Source: CAD feature listing. Evaluate the final solid. Frame: model axes, mm. A direction names the side the tool comes from. Give positions to 0.01 mm unless a question says otherwise; leave off trailing zeros. Write each loop counter-clockwise with the first axis right and the second up, starting at its lowest first coordinate (ties: lowest second). Pieces come first, ordered by that corner, then holes. Notation, with made-up numbers: M 26.5,-9.5 L 30.5,-9.5 A20 ccw 30.5,1.5 Z; hole C -39,38.5 d4. An arc over 180 degrees is marked long. Return JSON: item names as keys, results as strings.
```python
from build123d import *

# Parameters (mm, degrees)
SKETCH_1_W      = 14
SKETCH_1_H      = 14
EXTRUDE_1_DEPTH = 5
SKETCH_2_R      = 1.925
EXTRUDE_2_DEPTH = 2.8
CHAMFER_1_SIZE  = 0.5
SKETCH_3_W      = 15.6
SKETCH_3_H      = 15.6
EXTRUDE_3_DEPTH = 1
SKETCH_4_W      = 14
SKETCH_4_H      = 14
EXTRUDE_4_DEPTH = 5
EXTRUDE_5_DEPTH = 4.1


with BuildPart() as part:
    # 草图1 → 凸台-拉伸1 (new body)
    with BuildSketch(Plane(origin=(0, 0, 0), x_dir=(1, 0, 0), z_dir=(0, 1, 0))):
        with Locations((-2.892561983, 2.024793388)):
            Rectangle(SKETCH_1_W, SKETCH_1_H)
    extrude(amount=EXTRUDE_1_DEPTH)

    # 草图2 → 凸台-拉伸2 (add)
    with BuildSketch(Plane.XZ):
        with Locations(Location((-2.892561983, -2.024793388, 0), (0, 0, 270))):
            Circle(SKETCH_2_R)
    extrude(amount=EXTRUDE_2_DEPTH)

    # 倒角1
    chamfer_1_edges = [part.edges().sort_by_distance(p)[0] for p in [
        (-2.892561983, -2.8, -0.099793388),
    ]]
    chamfer(chamfer_1_edges, length=CHAMFER_1_SIZE)

    # 草图3 → 凸台-拉伸3 (add)
    with BuildSketch(Plane(origin=(0, 5, 0), x_dir=(1, 0, 0), z_dir=(0, 1, 0))):
        with Locations((-2.892561983, 2.024793388)):
            Rectangle(SKETCH_3_W, SKETCH_3_H)
    extrude(amount=EXTRUDE_3_DEPTH)

    # 草图4 → 凸台-拉伸4 (add)
    with BuildSketch(Plane(origin=(0, 6, 0), x_dir=(1, 0, 0), z_dir=(0, 1, 0))):
        with Locations((-2.892561983, 2.024793388)):
            Rectangle(SKETCH_4_W, SKETCH_4_H)
    extrude(amount=EXTRUDE_4_DEPTH)

    # 草图5 → 凸台-拉伸5 (add)
    with BuildSketch(Plane(origin=(0, 11, 0), x_dir=(1, 0, 0), z_dir=(0, 1, 0))):
        Polygon((-3.542561983, 2.674793388), (-3.542561983, 4.024793388), (-2.242561983, 4.024793388), (-2.242561983, 2.674793388), (-0.892561983, 2.674793388), (-0.892561983, 1.374793388), (-2.242561983, 1.374793388), (-2.242561983, 0.024793388), (-3.542561983, 0.024793388), (-3.542561983, 1.374793388), (-4.892561983, 1.374793388), (-4.892561983, 2.674793388), align=None)
    extrude(amount=EXTRUDE_5_DEPTH)


solid = part.part
```
1) Set-up query: faces 1 (the face through (4.107, 8, -2)), 2 (the face through (-3, 13, -0.025)), 3 (the face through (-4.893, 13, -2)), 4 (the face through (-3.543, 13, -1)), 5 (the face through (-4, 13, -2.675)). Return all of +Z, -Z, +X, -X, +Y, -Y with unobstructed straight access to the full face (end or side cutting, diameter ignored); none if empty.
Numbers:
{"face 1": "+Z, -Z, +X, +Y", "face 2": "+Z, +X, -X, +Y", "face 3": "+Z, -Z, -X, +Y", "face 4": "+Z, -X, +Y", "face 5": "-Z, -X, +Y"}
2) Line query: line 1 (Z direction, x = -0.75, y = 6.5); line 2 (X direction, y = 6.5, z = -1.25); line 3 (X direction, y = 14.5, z = -1.75). Output: solid intervals per line, ascending. Write a range as [from, to].
Numbers:
{"line 1": "z = [-9.02, 4.98]", "line 2": "x = [-9.89, 4.11]", "line 3": "x = [-4.89, -0.89]"}
3) Cut plane C-C, the plane y = 7.5. Return the cut outline in (x, z), then the cut area to 3 significant figures.
Numbers:
{"outline": "M -9.89,-9.02 L 4.11,-9.02 L 4.11,4.98 L -9.89,4.98 Z", "area": "196 mm²"}
4) Contact query for flat-ended pins moving along their axis: pin 1 Ø1.4 at (y, z) = (12, -2) entering from +X; pin 2 Ø1.1 at (y, z) = (13, -1) entering from -X; pin 3 Ø5 at (y, z) = (9.5, -4) entering from -X. Output: stop coordinate, or through.
Numbers:
{"pin 1": "stops at x = -0.89", "pin 2": "stops at x = -4.89", "pin 3": "stops at x = -9.89"}
5) Cut plane B-B, the plane z = 0.75. Return the cut outline in (x, y), then the cut area to 3 significant figures.
Numbers:
{"outline": "M -10.69,5 L -9.89,5 L -9.89,0 L 4.11,0 L 4.11,5 L 4.91,5 L 4.91,6 L 4.11,6 L 4.11,11 L -9.89,11 L -9.89,6 L -10.69,6 Z", "area": "156 mm²"}
6) Cut plane D-D, the plane y = -1.25. Return the cut outline in (x, z) (3 decimals).
Numbers:
{"outline": "C -2.893,-2.025 d3.85"}
7) Cut plane A-A, the plane x = -0.5. Return the cut outline in (y, z), then the cut area to 3 significant figures.
Numbers:
{"outline": "M 0,-9.02 L 5,-9.02 L 5,-9.82 L 6,-9.82 L 6,-9.02 L 11,-9.02 L 11,4.98 L 6,4.98 L 6,5.78 L 5,5.78 L 5,4.98 L 0,4.98 Z", "area": "156 mm²"}
